Geometry check sheet. Reference: the model listing, model coordinates, mm. Give positions to 0.01 mm unless a question says otherwise; leave off trailing zeros. Loops run counter-clockwise (first coordinate to the right, second up) from the corner with the lowest first, then second, coordinate; pieces in that order, holes last.
```python
from build123d import *

# Parameters (mm, degrees)
SKICA1_W                 = 350
SKICA1_H                 = 650
P_IDAT_VYSUNUT_M2_DEPTH  = 18
VETSI_W                  = 30
VETSI_H                  = 166
VETSI_H_2                = 30
ODEBRAT_VYSUNUT_M1_DEPTH = 15
P_IDAT_VYSUNUT_M3_DEPTH  = 5


with BuildPart() as part:
    # Skica1 → Přidat vysunutím2 (new body)
    with BuildSketch(Plane.XY):
        with Locations((175, 325)):
            Rectangle(SKICA1_W, SKICA1_H)
    extrude(amount=P_IDAT_VYSUNUT_M2_DEPTH)

    # vetsi → Odebrat vysunutím1 (cut)
    with BuildSketch(Plane.XY.offset(18)):
        with BuildLine():
            Line((65, 54), (65, 166))
            Line((65, 166), (50, 166))
            ThreePointArc((50, 166), (39.393398282, 170.393398282), (35, 181))
            Line((35, 181), (35, 54))
            ThreePointArc((35, 54), (50, 39), (65, 54))
        make_face()
        with BuildLine():
            ThreePointArc((65, 181), (60.606601718, 191.606601718), (50, 196))
            ThreePointArc((50, 196), (39.393398282, 191.606601718), (35, 181))
            ThreePointArc((35, 181), (39.393398282, 170.393398282), (50, 166))
            Line((50, 166), (65, 166))
            Line((65, 166), (65, 181))
        make_face()
        with BuildLine():
            Line((160, 166), (160, 196))
            Line((160, 196), (50, 196))
            ThreePointArc((50, 196), (60.606601718, 191.606601718), (65, 181))
            Line((65, 181), (65, 166))
            Line((65, 166), (160, 166))
        make_face()
        with Locations((175, 83)):
            Rectangle(VETSI_W, VETSI_H)
        with Locations((175, 181)):
            Rectangle(VETSI_W, VETSI_H_2)
        with BuildLine():
            Line((300, 196), (190, 196))
            Line((190, 196), (190, 166))
            Line((190, 166), (285, 166))
            Line((285, 166), (285, 181))
            ThreePointArc((285, 181), (289.393398282, 191.606601718), (300, 196))
        make_face()
        with BuildLine():
            ThreePointArc((315, 181), (310.606601718, 191.606601718), (300, 196))
            ThreePointArc((300, 196), (289.393398282, 191.606601718), (285, 181))
            Line((285, 181), (285, 166))
            Line((285, 166), (300, 166))
            ThreePointArc((300, 166), (310.606601718, 170.393398282), (315, 181))
        make_face()
        with BuildLine():
            Line((300, 166), (285, 166))
            Line((285, 166), (285, 54))
            ThreePointArc((285, 54), (300, 39), (315, 54))
            Line((315, 54), (315, 181))
            ThreePointArc((315, 181), (310.606601718, 170.393398282), (300, 166))
        make_face()
        with BuildLine():
            Line((190, 196), (190, 356))
            Line((190, 356), (175, 356))
            ThreePointArc((175, 356), (164.393398282, 360.393398282), (160, 371))
            Line((160, 371), (160, 196))
            Line((160, 196), (190, 196))
        make_face()
        with BuildLine():
            Line((282, 386), (190, 386))
            Line((190, 386), (190, 356))
            Line((190, 356), (282, 356))
            ThreePointArc((282, 356), (297, 371), (282, 386))
        make_face()
        with BuildLine():
            Line((190, 356), (190, 386))
            Line((190, 386), (175, 386))
            ThreePointArc((175, 386), (164.393398282, 381.606601718), (160, 371))
            ThreePointArc((160, 371), (164.393398282, 360.393398282), (175, 356))
            Line((175, 356), (190, 356))
        make_face()
        with BuildLine():
            Line((190, 386), (190, 407.000000086))
            ThreePointArc((190, 407.000000086), (185.606601748, 396.393398312), (175, 392))
            Line((175, 392), (160, 392))
            Line((160, 392), (160, 371))
            ThreePointArc((160, 371), (164.393398282, 381.606601718), (175, 386))
            Line((175, 386), (190, 386))
        make_face()
        with BuildLine():
            ThreePointArc((175, 392), (185.606601748, 396.393398312), (190, 407.000000086))
            ThreePointArc((190, 407.000000086), (185.606601688, 417.606601748), (175, 422))
            Line((175, 422), (160, 422))
            Line((160, 422), (160, 392))
            Line((160, 392), (175, 392))
        make_face()
        with BuildLine():
            Line((160, 392), (160, 422))
            Line((160, 422), (70, 422))
            ThreePointArc((70, 422), (55, 407), (70, 392))
            Line((70, 392), (160, 392))
        make_face()
        with BuildLine():
            Line((190, 407.000000086), (190, 520))
            Line((190, 520), (175, 520))
            ThreePointArc((175, 520), (164.393398282, 524.393398282), (160, 535))
            Line((160, 535), (160, 422))
            Line((160, 422), (175, 422))
            ThreePointArc((175, 422), (185.606601688, 417.606601748), (190, 407.000000086))
        make_face()
        with BuildLine():
            Line((190, 520), (190, 550))
            Line((190, 550), (175, 550))
            ThreePointArc((175, 550), (164.393398282, 545.606601718), (160, 535))
            ThreePointArc((160, 535), (164.393398282, 524.393398282), (175, 520))
            Line((175, 520), (190, 520))
        make_face()
        with BuildLine():
            Line((282, 550), (190, 550))
            Line((190, 550), (190, 520))
            Line((190, 520), (282, 520))
            ThreePointArc((282, 520), (297, 535), (282, 550))
        make_face()
        with BuildLine():
            Line((190, 550), (190, 600))
            ThreePointArc((190, 600), (185.606601718, 589.393398282), (175, 585))
            Line((175, 585), (160, 585))
            Line((160, 585), (160, 535))
            ThreePointArc((160, 535), (164.393398282, 545.606601718), (175, 550))
            Line((175, 550), (190, 550))
        make_face()
        with BuildLine():
            ThreePointArc((175, 585), (185.606601718, 589.393398282), (190, 600))
            ThreePointArc((190, 600), (185.606601718, 610.606601718), (175, 615))
            ThreePointArc((175, 615), (164.393398282, 610.606601718), (160, 600))
            Line((160, 600), (160, 585))
            Line((160, 585), (175, 585))
        make_face()
        with BuildLine():
            ThreePointArc((160, 600), (164.393398282, 610.606601718), (175, 615))
            Line((175, 615), (70, 615))
            ThreePointArc((70, 615), (55, 600), (70, 585))
            Line((70, 585), (160, 585))
            Line((160, 585), (160, 600))
        make_face()
    extrude(amount=-ODEBRAT_VYSUNUT_M1_DEPTH, mode=Mode.SUBTRACT)

    # mensi → Přidat vysunutím3 (add)
    with BuildSketch(Plane.XY.offset(18)):
        with BuildLine():
            ThreePointArc((175, 602.5), (176.767766953, 601.767766953), (177.5, 600))
            Line((177.5, 600), (177.5, 537.5))
            Line((177.5, 537.5), (282, 537.5))
            ThreePointArc((282, 537.5), (284.5, 535), (282, 532.5))
            Line((282, 532.5), (177.5, 532.5))
            Line((177.5, 532.5), (177.5, 406.999999943))
            Line((177.5, 406.999999943), (177.5, 373.5))
            Line((177.5, 373.5), (282, 373.5))
            ThreePointArc((282, 373.5), (284.5, 371), (282, 368.5))
            Line((282, 368.5), (177.5, 368.5))
            Line((177.5, 368.5), (177.5, 183.5))
            Line((177.5, 183.5), (300, 183.5))
            ThreePointArc((300, 183.5), (301.767766953, 182.767766953), (302.5, 181))
            Line((302.5, 181), (302.5, 54))
            ThreePointArc((302.5, 54), (300, 51.5), (297.5, 54))
            Line((297.5, 54), (297.5, 178.5))
            Line((297.5, 178.5), (177.5, 178.5))
            Line((177.5, 178.5), (177.5, 0))
            Line((177.5, 0), (350, 0))
            Line((350, 0), (350, 650))
            Line((350, 650), (0, 650))
            Line((0, 650), (0, 0))
            Line((0, 0), (172.5, 0))
            Line((172.5, 0), (172.5, 178.5))
            Line((172.5, 178.5), (52.5, 178.5))
            Line((52.5, 178.5), (52.5, 54))
            ThreePointArc((52.5, 54), (50, 51.5), (47.5, 54))
            Line((47.5, 54), (47.5, 181))
            ThreePointArc((47.5, 181), (48.232233047, 182.767766953), (50, 183.5))
            Line((50, 183.5), (172.5, 183.5))
            Line((172.5, 183.5), (172.5, 371))
            Line((172.5, 371), (172.5, 404.5))
            Line((172.5, 404.5), (70, 404.5))
            ThreePointArc((70, 404.5), (67.5, 407), (70, 409.5))
            Line((70, 409.5), (172.5, 409.5))
            Line((172.5, 409.5), (172.5, 535))
            Line((172.5, 535), (172.5, 597.5))
            Line((172.5, 597.5), (70, 597.5))
            ThreePointArc((70, 597.5), (67.5, 600), (70, 602.5))
            Line((70, 602.5), (175, 602.5))
        make_face()
    extrude(amount=-P_IDAT_VYSUNUT_M3_DEPTH)


solid = part.part
```
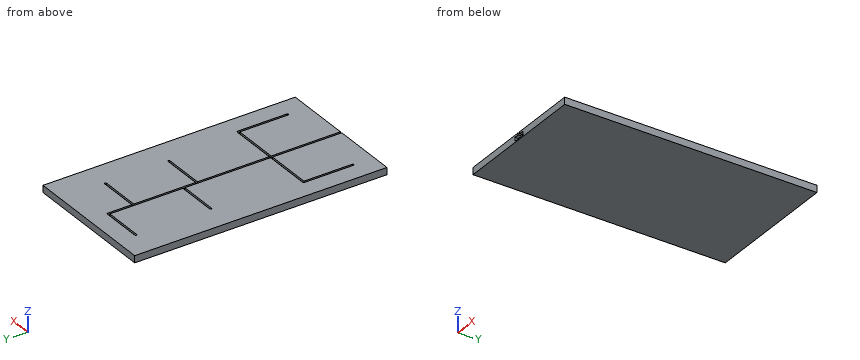
1) Sectioned sample at A-A on y = 556.5. Enter the section's corners in (x, z), plus the area to 4 significant figures.
2) Sectioned sample at B-B on x = 235. Enter the section's corners in (y, z), plus the area to 3 significant figures.
3) Scan lines: line 1 along Y through (x, z) = (79.5, 9); line 2 along Y through (x, z) = (146.5, 17.25); line 3 along X through (y, z) = (97, 14.75). Record each from-to range of solid material in increasing order.
Determined:
1. outline: (0, 0) - (350, 0) - (350, 18) - (177.5, 18) - (177.5, 13) - (190, 13) - (190, 3) - (160, 3) - (160, 13) - (172.5, 13) - (172.5, 18) - (0, 18) - close
1. area: 5,975 mm2
2. outline: (0, 0) - (650, 0) - (650, 18) - (537.5, 18) - (537.5, 13) - (550, 13) - (550, 3) - (520, 3) - (520, 13) - (532.5, 13) - (532.5, 18) - (373.5, 18) - (373.5, 13) - (386, 13) - (386, 3) - (356, 3) - (356, 13) - (368.5, 13) - (368.5, 18) - (183.5, 18) - (183.5, 13) - (196, 13) - (196, 3) - (166, 3) - (166, 13) - (178.5, 13) - (178.5, 18) - (0, 18) - close
2. area: 10,700 mm2
3. line 1: y = 0 to 166, 196 to 392, 422 to 585, 615 to 650
3. line 2: y = 0 to 178.5, 183.5 to 404.5, 409.5 to 597.5, 602.5 to 650
3. line 3: x = 0 to 47.5, 52.5 to 172.5, 177.5 to 297.5, 302.5 to 350
